Could you check a few things on this model? Use its own coordinates, in mm. A direction names the side the tool comes from. Round coordinates to 2 decimals unless told otherwise and drop trailing zeros. Write each loop counter-clockwise with the first axis right and the second up, starting at its lowest first coordinate (ties: lowest second). Pieces come first, ordered by that corner, then holes. Notation, with made-up numbers: M 77.5,33 L 121.5,33 A14 ccw 121.5,56 Z; hole C 51.5,70 d3. An arc over 180 degrees is marked long. One line per item, written item: value. Start each with the question number.
(1) If I drill on L1, parallel to Z at x = -41, y = -140.5; L2, parallel to Z at x = -56.5, y = -85; L3, parallel to X at y = -152.5, z = 51.5, over which ranges is the centre line in solid material (lowest first)?
(2) Thinking about a two-plate mould opening in Z: for faces 3 (the face through (-81.255, -81, 2)), 4 (the face through (-80.236, -81.345, 59)), 5 (the face through (-14, -81, 35.098)), which applies, released by +Z, released by -Z, zero draft, split by the parting line, or undercut?
(3) Which directions (+Z, -Z, +X, -X, +Y, -Y) give clear straight access to the entire face, cutting with the end or side of a thin tool? Please do faces 1 (the face through (-38.255, -81, -11)), 2 (the face through (-42, 0, 25)).
(4) I'm going to push flat-ended pins straight in: pin 1 Ø2 at (y, z) = (-66, -1) entering from +X; pin 2 Ø25 at (x, y) = (-12, -43) entering from -Z. Where does each tip first touch, or does it pass through?
(5) I want a section at C-C on z = 55. Please give me the cut outline in (x, y).
(6) I want a section at A-A on x = -32.5. Please give me the cut outline in (y, z).
(7) I want a section at B-B on z = 18.5. Please give me the cut outline in (x, y).
(8) I want a section at D-D on x = -46. Please give me the cut outline in (y, z).
```python
from build123d import *

# Parameters (mm, degrees)
F0_R     = 20.5
F1_DEPTH = 165


with BuildPart() as f1:
    # F0 (on Front) → F1 (new body)
    with BuildSketch(Plane.XZ):
        with BuildLine():
            Line((-81.255392, -55.654403), (-59.755392, -55.654403))
            Line((-59.755392, -55.654403), (-38.255392, -55.654403))
            Line((-38.255392, -55.654403), (-38.255392, 35.098321))
            Line((-38.255392, 35.098321), (11.744608, 35.098321))
            Line((11.744608, 35.098321), (11.744608, 84.345597))
            Line((11.744608, 84.345597), (-58.023451, 84.345597))
            add(Edge.make_bspline(
                [(-81.255392, 58.68857), (-81.255392, 69.632433), (-70.832212, 84.345597), (-58.023451, 84.345597)],
                knots=[0, 0, 0, 0, 34.612225, 34.612225, 34.612225, 34.612225], degree=3))
            Line((-81.255392, 58.68857), (-81.255392, -55.654403))
        make_face()
        with Locations((-59.755392, -29.901679)):
            Circle(F0_R, mode=Mode.SUBTRACT)
        with Locations((-59.755392, 14.098321)):
            Circle(F0_R, mode=Mode.SUBTRACT)
        with Locations((-59.755392, 58.098321)):
            Circle(F0_R, mode=Mode.SUBTRACT)
        with Locations((-15.755392, 58.098321)):
            Circle(F0_R, mode=Mode.SUBTRACT)
    extrude(amount=F1_DEPTH)


solid = f1.part
```
Found:
1. L1: z = -55.65 to -38.18, -21.63 to 5.82, 22.37 to 49.82, 66.37 to 84.35
1. L2: z = -55.65 to -50.14, -9.66 to -6.14, 34.34 to 37.86, 78.34 to 84.35
1. L3: x = -81.26 to -79.16, -40.35 to -35.16, 3.65 to 11.74
2. face 3: zero draft
2. face 4: undercut
2. face 5: released by -Z
3. face 1: -Z, +X, +Y, -Y
3. face 2: +Z, -Z, +X, -X, +Y
4. pin 1: stops at x = -38.26
4. pin 2: stops at z = 35.1
5. outline: M -81.26,-165 L -80.02,-165 L -80.02,0 L -81.26,0 Z; M -39.49,-165 L -36.02,-165 L -36.02,0 L -39.49,0 Z; M 4.51,-165 L 11.74,-165 L 11.74,0 L 4.51,0 Z
6. outline: M -165,35.1 L 0,35.1 L 0,46.27 L -165,46.27 Z; M -165,69.92 L 0,69.92 L 0,84.35 L -165,84.35 Z
7. outline: M -81.26,-165 L -79.78,-165 L -79.78,0 L -81.26,0 Z; M -39.73,-165 L -38.26,-165 L -38.26,0 L -39.73,0 Z
8. outline: M -165,-55.65 L 0,-55.65 L 0,-45.1 L -165,-45.1 Z; M -165,-14.7 L 0,-14.7 L 0,-1.1 L -165,-1.1 Z; M -165,29.3 L 0,29.3 L 0,42.9 L -165,42.9 Z; M -165,73.3 L 0,73.3 L 0,84.35 L -165,84.35 Z
